For this review, take the finished solid that the model builds, in its own axes (mm). A direction names the side the tool comes from. Coordinates: 2 decimals unless noted, no trailing zeros. Write each loop counter-clockwise with the first axis right and the second up, starting at its lowest first coordinate (ties: lowest second). Pieces come first, ordered by that corner, then holes. Notation, with made-up numbers: M -33.75,10 L -6.75,10 A23 ccw -6.75,44 Z; hole C 67.25,78 d7. An arc over 180 degrees is marked long. Return JSON: item names as keys, results as strings.
Autodesk Fusion 360 part; units mm, degrees
sketch "Sketch1" plane through (0, 0, 0) normal (0, 1, 0) x (1, 0, 0)
  line L0 (0, 0) -> (18, 0)
  line L1 (0, 0) -> (-18, 0)
  line L2 (25, 7) -> (25, 22)
  line L3 (-25, 7) -> (-25, 22)
  line L4 (25, 22) -> (31, 22)
  line L5 (-25, 22) -> (-31, 22)
  line L6 (0, 0) -> (0, -27.55) construction
  line L7 (0, -27.55) -> (35, -27.55)
  line L8 (0, -27.55) -> (-35, -27.55)
  line L9 (31, 22) -> (31, 7)
  line L10 (-31, 22) -> (-31, 7)
  line L11 (-35, -27.55) -> (-31, 7)
  line L12 (35, -27.55) -> (31, 7)
  arc A0 (-25, 7) -> (-18, 0) centre (-18, 7) ccw
  arc A1 (18, 0) -> (25, 7) centre (18, 7) ccw
  point P0 (25, 0)
  point P1 (-25, 0)
  dimension "d5" = 25
  dimension "d6" = 25
  dimension "d7" = 22
  dimension "d8" = 22
  dimension "d9" = 6
  dimension "d10" = 6
  dimension "d11" = 27.55
  dimension "d12" = 35
  dimension "d13" = 35
  dimension "d14" = 15
  dimension "d15" = 15
  dimension "d16" = 7
  dimension "d17" = 7
extrude "Extrude1" add sketch "Sketch1" along normal blind 40
sketch "Sketch2" plane through (0, 0, 27.55) normal (0, 0, 1) x (-1, 0, 0)
  line L0 (35, 0) -> (-35, 0)
  line L1 (-35, 0) -> (-35, -40)
  line L2 (-35, -40) -> (35, -40)
  line L3 (35, -40) -> (35, 0)
  line L4 (0, -40) -> (0, -32.5) construction
  line L5 (0, 0) -> (0, -7.5) construction
  line L6 (0, -32.5) -> (-15, -32.5) construction
  line L7 (0, -32.5) -> (15, -32.5) construction
  circle A0 centre (15, -32.5) radius 3.5
  circle A1 centre (15, -32.5) radius 5.25
  circle A2 centre (-15, -32.5) radius 3.5
  circle A3 centre (-15, -32.5) radius 5.25
  circle A4 centre (0, -7.5) radius 3.5
  circle A5 centre (0, -7.5) radius 5.25
  line L8 (-35, 0) -> (-27, 0) construction
  line L9 (-27, 0) -> (-27, -7.5) construction
  line L10 (-27, -7.5) -> (-35, -7.5) construction
  line L11 (-35, -7.5) -> (-35, 0) construction
  line L12 (35, 0) -> (27, 0) construction
  line L13 (27, 0) -> (27, -7.5) construction
  line L14 (27, -7.5) -> (35, -7.5) construction
  line L15 (35, -7.5) -> (35, 0) construction
  line L16 (-27, -7.5) -> (-27, -22.5) construction
  line L17 (27, -7.5) -> (27, -22.5) construction
  circle A6 centre (-27, -22.5) radius 2.9
  circle A7 centre (-27, -7.5) radius 2.9
  circle A8 centre (27, -7.5) radius 2.9
  circle A9 centre (27, -22.5) radius 2.9
  dimension "d20" = 7.5
  dimension "d21" = 7.5
  dimension "d22" = 15
  dimension "d23" = 15
  dimension "d24" = 7
  dimension "d25" = 10.5
  dimension "d26" = 7
  dimension "d27" = 10.5
  dimension "d28" = 7
  dimension "d29" = 10.5
  dimension "d30" = 8
  dimension "d31" = 7.5
  dimension "d32" = 8
  dimension "d33" = 7.5
  dimension "d34" = 15
  dimension "d35" = 15
  dimension "d36" = 5.8
  dimension "d37" = 5.8
  dimension "d38" = 5.8
  dimension "d39" = 5.8
extrude "Extrude4" cut sketch "Sketch2" against normal through all contours A0 | A2 | A4
extrude "Extrude3" cut sketch "Sketch2" against normal blind 7 contours A1 | A3 | A5
extrude "Extrude2" cut sketch "Sketch2" against normal up to surface (27.55 mm away) contours A6 | A7 | A8 | A9
chamfer "Chamfer1" distance 2 angle 45 8 edges at (33, 0, 10.275) (31, 0, -14.5) (-31, 0, -14.5) (-33, 0, 10.275) (-31, 40, -14.5) (-33, 40, 10.275) (33, 40, 10.275) (31, 40, -14.5)
chamfer "Chamfer2" distance 2 angle 45 2 edges at (-31, 20, -22) (31, 20, -22)
equation "steelRadius = 7 mm"
equation "steelNarrow = 50 mm"
equation "d5 = steelNarrow / 2"
equation "d6 = steelNarrow / 2"
equation "d16 = steelRadius"
equation "d17 = steelRadius"
1. For faces 4 (the face through (-30, 1, -15)), 5 (the face through (-30, 39, -15)), 6 (the face through (4, 7, 20.55)), 7 (the face through (31, 20, -14)), 8 (the face through (-31, 20, -14)), list the 3-axis set-ups (+Z, -Z, +X, -X, +Y, -Y) from which the entire face can be reached by the end or side of a thin tool; tool diameter is ignored.
Checks:
{"face 4": "-Z, -X, -Y", "face 5": "-Z, -X, +Y", "face 6": "+Z", "face 7": "-Z, +X, +Y, -Y", "face 8": "-Z, -X, +Y, -Y"}
2. We need section C-C (z = -16). State the section outline as (x, y) points.
Checks:
{"outline": "M -31,2 L -29,0 L -25,0 L -25,40 L -29,40 L -31,38 Z; M 25,0 L 29,0 L 31,2 L 31,38 L 29,40 L 25,40 Z"}
3. Draft analysis for pull direction Y (two halves, no side actions). For faces 1 (the face through (27, 22, 0)), 2 (the face through (33.03, 19.75, 10.52)), 3 (the face through (-32.04, 38.99, 10.57)), state which applies: +Y half, -Y half, draft (parallel to the pull), parting line (faces both ways), or undercut.
Checks:
{"face 1": "undercut", "face 2": "draft", "face 3": "+Y half"}
4. Clearance check with flat-ended pins moving along their axes: pin 1 Ø1 at (x, y) = (-2, 34.5) entering from -Z; pin 2 Ø1.7 at (x, y) = (-27, 23) entering from +Z; pin 3 Ø10.5 at (y, z) = (17.5, -11) entering from +X. State where each tip first meets the part, or that it passes through.
Checks:
{"pin 1": "z = 0", "pin 2": "z = 0", "pin 3": "x = 31.14"}
5. We need section D-D (y = 22.5). State the section outline as (x, z) points.
Checks:
{"outline": "M -35,27.55 L -31,-7 L -31,-20 L -29,-22 L -25,-22 L -25,-7 A7 cw -18,0 L 18,0 A7 cw 25,-7 L 25,-22 L 29,-22 L 31,-20 L 31,-7 L 35,27.55 L 29.9,27.55 L 29.9,0 L 24.1,0 L 24.1,27.55 L -24.1,27.55 L -24.1,0 L -29.9,0 L -29.9,27.55 Z"}
6. Wall thickness on L1, parallel to Y at x = -27, z = 20; L2, parallel to X at y = 6, z = -14.5; L3, parallel to Y at x = 0, z = 24: over which ranges is each line inside the solid? List them lowest first. Write a range as from..to.
Checks:
{"L1": "0..4.6, 10.4..19.6, 25.4..40", "L2": "-31..-25, 25..31", "L3": "0..2.25, 12.75..40"}
7. We need section A-A (x = 15). State the section outline as (y, z) points, plus the area to 3 significant figures.
Checks:
{"outline": "M 0,0 L 29,0 L 29,20.55 L 27.25,20.55 L 27.25,27.55 L 0,27.55 Z; M 36,0 L 40,0 L 40,27.55 L 37.75,27.55 L 37.75,20.55 L 36,20.55 Z", "area": "885 mm2"}
